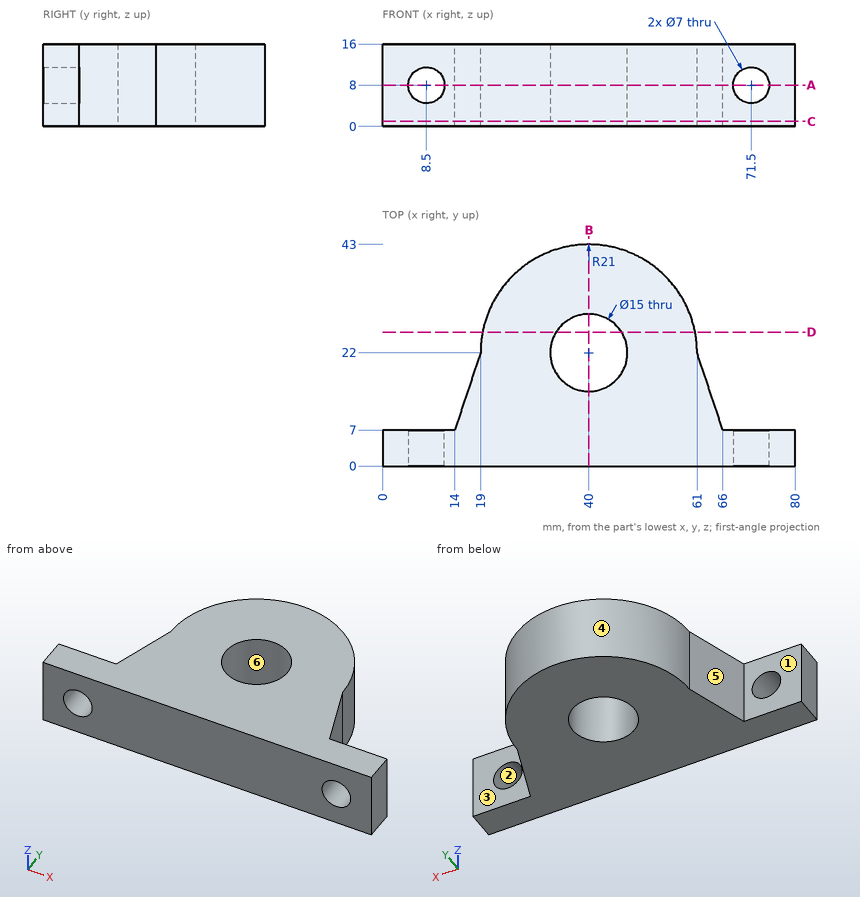
Verification items for this drawing (mm, ordinates from the low corner). A direction names the side the tool comes from. Give positions to 0.01 mm unless a question says otherwise; leave off trailing zeros. Loops run counter-clockwise (first coordinate to the right, second up) from the corner with the lowest first, then second, coordinate; pieces in that order, holes last. Notation, with made-up numbers: M 48,73 L 104,73 A35 cw 104,108 Z; hole C 45.5,64.5 d9. An arc over 180 degrees is marked long. Answer as a JSON object with one key per item and string values. Group by question number.
Q1. Access from +Z, -Z, +X, -X, +Y, -Y to the whole of each face (thin tool, end or side, straight path). Record for the marked faces 1, 2 and 3.
Q2. Cross-section at B-B on x = 40. Record the cut outline in (y, z).
Q3. Go/stop test with flat-tipped pins: P1, Ø8, axis at x = 44, z = 4.5, coming from the +Y side; P2, Ø10, axis at x = 41.5, y = 10, coming from the -Z side; P3, Ø8, axis at x = 71.5, z = 8, coming from the +Y side; P4, Ø1, axis at y = 38.5, z = 9, coming from the +X side. Record where each tip stops, or that it passes through.
Q4. Cross-section at A-A on z = 8. Record the cut outline in (x, y).
Q5. Release check for a two-part mould opening along X. For the marked faces 4, 5 and 6 record: released by +X, released by -X, zero draft, split by the parting line, or undercut.
Q6. Material ranges on line 1 along Z through (x, y) = (71.5, 5.5); line 2 along X through (y, z) = (5, 5.5); line 3 along X through (y, z) = (22.5, 13.25), recorded low to high. Write a range as [from, to].
Q7. Cross-section at C-C on z = 1. Record the cut outline in (x, y), then the cut area to 3 significant figures.
Q8. Cross-section at D-D on y = 26. Record the cut outline in (x, z), then the cut area to 3 significant figures.
Evaluation:
{
 "1": {"face 1": "+Z, -Z, -X, +Y", "face 2": "+Y, -Y", "face 3": "+Z, -Z, +X, +Y"},
 "2": {"outline": "M 0,0 L 14.5,0 L 14.5,16 L 0,16 Z; M 29.5,0 L 43,0 L 43,16 L 29.5,16 Z"},
 "3": {"P1": "stops at y = 43", "P2": "stops at z = 0", "P3": "stops at y = 7", "P4": "stops at x = 53.6"},
 "4": {"outline": "M 0,0 L 5,0 L 5,7 L 0,7 Z; M 12,0 L 68,0 L 68,7 L 66,7 L 61,22 A21 ccw 19,22 L 14,7 L 12,7 Z; M 75,0 L 80,0 L 80,7 L 75,7 Z; hole C 40,22 d15"},
 "5": {"face 4": "split by the parting line", "face 5": "released by -X", "face 6": "undercut"},
 "6": {"line 1": "z = [0, 4.5], [11.5, 16]", "line 2": "x = [0, 6.05], [10.95, 69.05], [73.95, 80]", "line 3": "x = [19.01, 32.52], [47.48, 60.99]"},
 "7": {"outline": "M 0,0 L 80,0 L 80,7 L 66,7 L 61,22 A21 ccw 19,22 L 14,7 L 0,7 Z; hole C 40,22 d15", "area": "1,780 mm2"},
 "8": {"outline": "M 19.38,0 L 33.66,0 L 33.66,16 L 19.38,16 Z; M 46.34,0 L 60.62,0 L 60.62,16 L 46.34,16 Z", "area": "457 mm2"}
}
